from build123d import *

# Parameters (mm, degrees)
ESQUISSE1_W        = 50
ESQUISSE1_H        = 40
BOSS_EXTRU_1_DEPTH = 30
BOSS_EXTRU_2_DEPTH = 200


with BuildPart() as part:
    # Esquisse1 → Boss.-Extru.1 (new body)
    with BuildSketch(Plane(origin=(0, 0, 0), x_dir=(1, 0, 0), z_dir=(0, 1, 0))):
        Rectangle(ESQUISSE1_W, ESQUISSE1_H)
    extrude(amount=BOSS_EXTRU_1_DEPTH)

    # Esquisse2 → Boss.-Extru.2 (add)
    with BuildSketch(Plane(origin=(0, 30, 0), x_dir=(1, 0, 0), z_dir=(0, 1, 0))):
        Polygon((-10, -20), (10, -20), (10, -18), (5, -18), (5, -10), (10, -10), (10, -8), (-10, -8), (-10, -10), (-5, -10), (-5, -18), (-10, -18), align=None)
    extrude(amount=BOSS_EXTRU_2_DEPTH)


solid = part.part
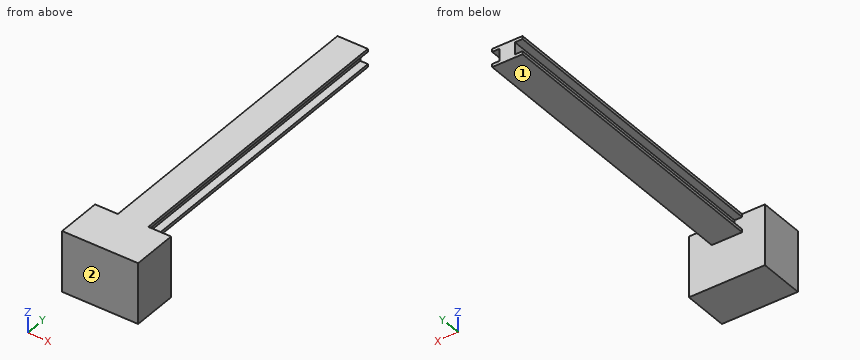
CAD build for the part. Positions are in the model's coordinates, mm. Face numbers are marked on the shaded views. A direction names the side the tool comes from. Round coordinates to 2 decimals unless told otherwise and drop trailing zeros. Loops run counter-clockwise (first coordinate to the right, second up) from the corner with the lowest first, then second, coordinate; pieces in that order, holes last.
(1) Cut at B-B (y = 198). Give the cut face in (x, z), plus the area to 3 significant figures.
(2) Wall check: line 1 along Z through (x, y) = (-6, 135); line 2 along Y through (x, z) = (-20, -12.5); line 3 along X through (y, z) = (154.5, 14.5). Give the ranges that are in metal, low to high.
(3) Drop flat-ended pins along their axis: pin 1 (2 mm diameter, centred on x = 11.5, z = 9, fed in from +Y); pin 2 (4 mm diameter, centred on x = 6.5, y = 146, fed in from -Z); pin 3 (6.5 mm diameter, centred on y = 134, z = 14, fed in from -X). Give the stop position or say it passes through.
(4) Cut at D-D (x = -17). Give the cut face in (y, z), plus the area to 3 significant figures.
(5) Cut at A-A (z = 15). Give the cut face in (x, y), plus the area to 3 significant figures.
(6) Which spindle directions (+Z, -Z, +X, -X, +Y, -Y) get a long thin tool onto all of the face, cutting with end or side? Do the marked faces 1 and 2. Say none if no direction does.
(7) Cut at C-C (x = 1). Give the cut face in (y, z).
Findings below:
1. outline: (-10, 8) - (10, 8) - (10, 10) - (5, 10) - (5, 18) - (10, 18) - (10, 20) - (-10, 20) - (-10, 18) - (-5, 18) - (-5, 10) - (-10, 10) - close
1. area: 160 mm2
2. line 1: z = 8 to 10, 18 to 20
2. line 2: y = 0 to 30
2. line 3: x = -5 to 5
3. pin 1: stops at y = 30
3. pin 2: stops at z = 8
3. pin 3: stops at x = -5
4. outline: (0, -20) - (30, -20) - (30, 20) - (0, 20) - close
4. area: 1,200 mm2
5. outline: (-25, 0) - (25, 0) - (25, 30) - (5, 30) - (5, 230) - (-5, 230) - (-5, 30) - (-25, 30) - close
5. area: 3,500 mm2
6. face 1: -Z, +X, -X, +Y
6. face 2: +Z, -Z, +X, -X, -Y
7. outline: (0, -20) - (30, -20) - (30, 8) - (230, 8) - (230, 20) - (0, 20) - close
